```python
from build123d import *

# Parameters (mm, degrees)
EXTRUDE_THIN1_DEPTH     = 8
SHELL4_T                = -1
CUT_EXTRUDE_THIN1_DEPTH = 8


with BuildPart() as part:
    # Sketch1 → Extrude-Thin1 (new body)
    with BuildSketch(Plane(origin=(0, 0, 0), x_dir=(0, 1, 0), z_dir=(0, 0, 1))):
        Polygon((2.5, 0), (2.5, 2.556624327), (9.910254038, 6.834936491), (7.410254038, 11.165063509), (-2.5, 5.443375673), (-2.5, 0), align=None)
    extrude_thin1 = extrude(amount=EXTRUDE_THIN1_DEPTH)

    # Mirror3: Extrude-Thin1 across plane
    add(extrude_thin1.mirror(Plane.ZX))

    # Shell4
    shell4_openings = [part.faces().sort_by_distance(p)[0] for p in [
        (-5.923522884, 0, 8),
        (0, 0, 4),
    ]]
    offset(amount=SHELL4_T, openings=shell4_openings, kind=Kind.INTERSECTION)

    # Sketch5 → Cut-Extrude-Thin1 (cut)
    with BuildSketch(Plane(origin=(-6, 10.392304845, 0), x_dir=(-0.8660254037844398, -0.49999999999999806, 0), z_dir=(-0.499999999999998, 0.8660254037844397, 0))):
        with BuildLine():
            ThreePointArc((2.10203265, 6.155172414), (2.964101615, 4), (2.10203265, 1.844827586))
            Line((2.10203265, 1.844827586), (2.826170581, 1.155172414))
            ThreePointArc((2.826170581, 1.155172414), (3.964101615, 4), (2.826170581, 6.844827586))
            Line((2.826170581, 6.844827586), (2.10203265, 6.155172414))
        make_face()
    cut_extrude_thin1 = extrude(amount=-CUT_EXTRUDE_THIN1_DEPTH, mode=Mode.SUBTRACT)

    # Mirror4: Cut-Extrude-Thin1 across plane
    add(cut_extrude_thin1.mirror(Plane.ZX), mode=Mode.SUBTRACT)


solid = part.part
```
Part model, mm, in its own coordinate system. A direction names the side the tool comes from. Give positions to 0.01 mm unless a question says otherwise; leave off trailing zeros. Loops run counter-clockwise (first coordinate to the right, second up) from the corner with the lowest first, then second, coordinate; pieces in that order, holes last. Notation, with made-up numbers: M -10.75,58 L 33.25,58 A23 cw 33.25,81 Z; hole C -26.75,-35.5 d1. An arc over 180 degrees is marked long. Return JSON: item names as keys, results as strings.
1) Flat gauge pins, fed straight in: pin 1 Ø1 at (x, y) = (-3.5, -6.5) entering from -Z; pin 2 Ø2.5 at (x, z) = (-1.5, 4) entering from -Y; pin 3 Ø2 at (x, y) = (-3, -3.5) entering from +Z; pin 4 Ø2 at (x, z) = (-2, 4) entering from -Y. Where does each tip first touch, or does it go through?
Calculated:
{"pin 1": "passes through", "pin 2": "stops at y = -2.83", "pin 3": "stops at z = 8", "pin 4": "stops at y = -3.27"}
2) Saw through at C-C, the plane z = 4.25. List the corners of the cut face in (x, y).
Calculated:
{"outline": "M -11.17,-7.41 L -9.43,-8.41 L -8.93,-7.55 L -9.8,-7.04 L -5.73,0 L -9.8,7.04 L -8.93,7.55 L -9.43,8.41 L -11.17,7.41 L -6.89,0 Z; M -8.56,-8.92 L -6.83,-9.91 L -2.56,-2.5 L 0,-2.5 L 0,-1.5 L -3.13,-1.5 L -7.2,-8.54 L -8.06,-8.05 Z; M -8.56,8.92 L -8.06,8.05 L -7.2,8.54 L -3.13,1.5 L 0,1.5 L 0,2.5 L -2.56,2.5 L -6.83,9.91 Z"}
3) 3-axis set-ups, long thin cutter, end or side, ignore diameter. For faces 1 (the face through (-9.932, 8.122, 3.944)), 2 (the face through (-1, -2.5, 4)), 3 (the face through (-8.32, 8.48, 4.03)), 4 (the face through (-7.794, 3.571, 4.451)), 5 (the face through (-4.666, 6.153, 3.944)): which of +Z, -Z, +X, -X, +Y, -Y reach the whole face in a straight line?
Calculated:
{"face 1": "+Z, -Z, -X, +Y", "face 2": "+Z, -Z, +X, -Y", "face 3": "none", "face 4": "+Z", "face 5": "+Z, -Z, +X, +Y"}
4) Drill centre lines: line 1 (Y direction, x = -0.75, z = 4); line 2 (Y direction, x = -9, z = 7.75); line 3 (Y direction, x = -7.5, z = 6). Where is each one in solid material? Low to high.
Calculated:
{"line 1": "y = -2.5 to -1.5, 1.5 to 2.5", "line 2": "y = -8.66 to -7.51, -5.66 to -3.66, 3.66 to 5.66, 7.51 to 8.66", "line 3": "y = -9.53 to -8.51, -3.06 to -1.06, 1.06 to 3.06, 8.51 to 9.53"}
5) Pull direction X, two halves, no side cores. Call faces 6 (the face through (-1, 2.5, 4)), 7 (the face through (-9.186, -7.983, 3.956)), 8 (the face through (-4.666, -6.153, 3.944)): released by +X, released by -X, zero draft, split by the parting line, or undercut.
Calculated:
{"face 6": "zero draft", "face 7": "undercut", "face 8": "released by +X"}
6) Saw through at D-D, the plane y = -4.25. List the corners of the cut face in (x, z).
Calculated:
{"outline": "M -9.34,0 L -3.57,0 L -3.57,8 L -4.72,8 L -4.72,1 L -8.19,1 L -8.19,8 L -9.34,8 Z"}
7) Saw through at B-B, the plane z = 7.25. List the corners of the cut face in (x, y), then the cut area to 3 significant figures.
Calculated:
{"outline": "M -11.17,-7.41 L -6.83,-9.91 L -2.56,-2.5 L 0,-2.5 L 0,-1.5 L -3.13,-1.5 L -7.2,-8.54 L -9.8,-7.04 L -5.73,0 L -9.8,7.04 L -7.2,8.54 L -3.13,1.5 L 0,1.5 L 0,2.5 L -2.56,2.5 L -6.83,9.91 L -11.17,7.41 L -6.89,0 Z", "area": "47.1 mm2"}
8) Saw through at A-A, the plane x = -4. List the corners of the cut face in (y, z).
Calculated:
{"outline": "M -5,0 L 5,0 L 5,8 L 3,8 L 3,1 L -3,1 L -3,8 L -5,8 Z"}
